Read the model definition and answer for the solid it produces. Units are mm, in the model's axes. Face numbers are marked on the shaded views. A direction names the side the tool comes from. Coordinates: 2 decimals unless noted, no trailing zeros. Loops run counter-clockwise (first coordinate to the right, second up) from the corner with the lowest first, then second, coordinate; pieces in that order, holes last.
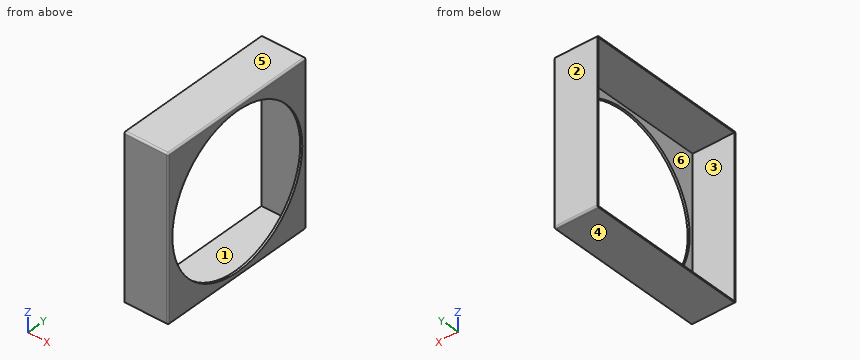
Autodesk Inventor part; units mm, degrees
ref_plane "YZ Plane" through (0, 0, 0) normal (1, 0, 0) x (0, 1, 0)
ref_plane "XZ Plane" through (0, 0, 0) normal (0, 1, 0) x (-1, 0, 0)
ref_plane "XY Plane" through (0, 0, 0) normal (0, 0, 1) x (1, 0, 0)
sketch "Sketch1" plane through (0, 0, 0) normal (1, 0, 0) x (0, 1, 0)
  circle A0 centre (0, 0) radius 139.7
  line L0 (0, -139.7) -> (0, -146.05)
  line L1 (-139.7, 0) -> (-146.05, 0)
  line L2 (146.05, 0) -> (146.05, -146.05)
  line L3 (146.05, -146.05) -> (-146.05, -146.05)
  line L4 (-146.05, -146.05) -> (-146.05, 146.05)
  line L5 (-146.05, 146.05) -> (146.05, 146.05)
  line L6 (146.05, 146.05) -> (146.05, 0)
  dimension "d1" = 279.4
sketch "Sketch2" plane through (0, 0, 0) normal (0, 0, 1) x (1, 0, 0)
  point P0 (0, 0)
extrude "Extrusion1" add sketch "Sketch1" along normal blind 3.81 contours A0 L1 L4 L5 L6 L2 L3 L0 | A0 L0 L3 L4 L1
sketch "Sketch3" plane through (0, -146.05, 146.05) normal (0, 0, 1) x (1, 0, 0)
  line L0 (0, 292.1) -> (0, 0)
  line L1 (3.81, 292.1) -> (-76.2, 292.1)
  line L2 (-76.2, 292.1) -> (-76.2, 0)
  line L3 (-76.2, 0) -> (3.81, 0)
  point P0 (0, 146.05)
  dimension "d12" = 80.01
extrude "Extrusion3" add sketch "Sketch3" along normal blind 2.54
sketch "Sketch4" plane through (3.81, -146.05, -146.05) normal (0, -1, 0) x (1, 0, 0)
  line L0 (-3.81, 292.1) -> (0, 292.1)
  line L1 (-3.81, 292.1) -> (-80.01, 292.1)
  line L2 (-3.81, 292.1) -> (-80.01, 292.1)
  line L3 (-3.81, 292.1) -> (-3.81, 0)
  line L4 (-3.81, 0) -> (-80.01, 0)
  line L5 (-80.01, 0) -> (-80.01, 292.1)
  point P0 (-3.81, 146.05)
  dimension "d15" = 76.2
extrude "Extrusion4" add sketch "Sketch4" along normal blind 2.54
sketch "Sketch6" plane through (3.81, -146.05, -146.05) normal (0, 0, -1) x (-1, 0, 0)
  line L0 (80.01, 0) -> (3.81, 0)
  line L1 (3.81, 0) -> (80.01, 0)
  line L2 (80.01, 292.1) -> (80.01, 0)
  line L3 (80.01, 0) -> (80.01, 292.1)
  line L4 (80.01, 292.1) -> (3.81, 292.1)
  line L5 (3.81, 292.1) -> (3.81, 0)
  line L6 (3.81, 6.35) -> (3.81, 285.75)
  point P0 (3.81, 146.05)
extrude "Extrusion5" add sketch "Sketch6" along normal blind 2.54
sketch "Sketch7" plane through (3.81, 146.05, 146.05) normal (0, 1, 0) x (1, 0, 0)
  line L0 (-3.81, 292.1) -> (0, 292.1)
  line L1 (-3.81, 292.1) -> (-80.01, 292.1)
  line L2 (-80.01, 292.1) -> (-80.01, 0)
  line L3 (-80.01, 0) -> (-3.81, 0)
  line L4 (-3.81, 292.1) -> (-3.81, 0)
  point P0 (-3.81, 146.05)
extrude "Extrusion6" add sketch "Sketch7" along normal blind 2.54
sketch "Sketch21" plane through (-76.2, -148.59, -146.05) normal (-1, 0, 0) x (0, 0, 1)
  line L0 (0, 0) -> (-2.54, 0)
  line L1 (-2.54, 0) -> (-2.54, 2.54)
  line L2 (0, 2.54) -> (-2.54, 2.54)
  line L3 (-2.54, 2.54) -> (0, 2.54)
  line L4 (0, 2.54) -> (0, 0)
  line L5 (0, 2.54) -> (0, 0)
  point P0 (146.05, 148.59)
extrude "Extrusion16" add sketch "Sketch21" against normal up to surface (76.2 mm away)
sketch "Sketch22" plane through (3.81, 148.59, 146.05) normal (0, 1, 0) x (1, 0, 0)
  line L0 (-3.81, 0) -> (-3.81, 294.64)
  line L1 (-80.01, 292.1) -> (-3.81, 292.1)
  line L2 (-3.81, 294.64) -> (-3.81, 292.1)
  line L3 (0, 292.1) -> (0, 0)
  line L4 (-3.81, 292.1) -> (0, 292.1)
  line L5 (0, 292.1) -> (0, 294.64)
  line L6 (0, 294.64) -> (-3.81, 294.64)
  point P0 (-3.81, 146.05)
extrude "Extrusion17" add sketch "Sketch22" against normal up to surface (297.18 mm away)
sketch "Sketch23" plane through (-76.2, -146.05, -146.05) normal (-1, 0, 0) x (0, 0, 1)
  line L0 (0, 292.1) -> (-2.54, 292.1)
  line L1 (-2.54, 292.1) -> (0, 292.1)
  line L2 (292.1, 294.64) -> (0, 294.64)
  line L3 (0, 292.1) -> (0, 294.64)
  line L4 (-2.54, 294.64) -> (-2.54, -2.54)
  line L5 (0, 294.64) -> (-2.54, 294.64)
  line L6 (-2.54, 294.64) -> (-2.54, 292.1)
  point P0 (146.05, 146.05)
extrude "Extrusion18" add sketch "Sketch23" against normal up to surface (76.2 mm away)
sketch "Sketch26" plane through (0, -146.05, 148.59) normal (0, 0, 1) x (1, 0, 0)
  line L0 (0, 292.1) -> (3.81, 292.1)
  line L1 (3.81, 292.1) -> (0, 292.1)
  line L2 (0, 292.1) -> (0, 294.64)
  line L3 (0, 292.1) -> (0, 294.64)
  line L4 (0, 294.64) -> (3.81, 294.64)
  line L5 (3.81, 294.64) -> (3.81, 292.1)
  point P0 (0, 146.05)
extrude "Extrusion20" add sketch "Sketch26" against normal up to surface (294.64 mm away)
sketch "Sketch27" plane through (0, -146.05, 148.59) normal (0, 0, 1) x (1, 0, 0)
  line L0 (0, 0) -> (3.81, 0)
  line L1 (3.81, 0) -> (0, 0)
  line L2 (0, 0) -> (0, -2.54)
  line L3 (0, 0) -> (0, -2.54)
  line L4 (0, -2.54) -> (3.81, -2.54)
  line L5 (0, -2.54) -> (3.81, -2.54)
  line L6 (3.81, 0) -> (3.81, -2.54)
  line L7 (3.81, -2.54) -> (3.81, 0)
  point P0 (0, 146.05)
extrude "Extrusion21" add sketch "Sketch27" against normal up to surface (294.64 mm away)
sketch "Sketch28" plane through (0, 146.05, 148.59) normal (0, -1, 0) x (1, 0, 0)
  line L0 (3.81, 0) -> (3.81, -2.54)
  line L1 (3.81, 0) -> (3.81, -2.54)
  line L2 (3.81, -2.54) -> (0, -2.54)
  line L3 (0, -2.54) -> (0, 0)
  line L4 (0, 0) -> (3.81, 0)
  point P0 (0, -148.59)
extrude "Extrusion22" add sketch "Sketch28" along normal up to surface (292.1 mm away)
sketch "Sketch29" plane through (-76.2, -146.05, -146.05) normal (-1, 0, 0) x (0, 0, 1)
  line L0 (292.1, 292.1) -> (294.64, 292.1)
  line L1 (294.64, 292.1) -> (292.1, 292.1)
  line L2 (292.1, 292.1) -> (292.1, 294.64)
  line L3 (292.1, 292.1) -> (292.1, 294.64)
  line L4 (294.64, 294.64) -> (294.64, 292.1)
  line L5 (292.1, 294.64) -> (294.64, 294.64)
  line L6 (294.64, 294.64) -> (294.64, 292.1)
  point P0 (146.05, 146.05)
extrude "Extrusion23" add sketch "Sketch29" against normal up to surface (76.2 mm away)
sketch "Sketch30" plane through (-76.2, -146.05, -146.05) normal (-1, 0, 0) x (0, 0, 1)
  line L0 (292.1, 0) -> (0, 0)
  line L1 (292.1, 0) -> (292.1, -2.54)
  line L2 (294.64, -2.54) -> (-2.54, -2.54)
  line L3 (294.64, -2.54) -> (294.64, 0)
  line L4 (294.64, -2.54) -> (294.64, 294.64)
  line L5 (292.1, 0) -> (294.64, 0)
  line L6 (292.1, 0) -> (292.1, -2.54)
  line L7 (292.1, -2.54) -> (294.64, -2.54)
  point P0 (146.05, 146.05)
extrude "Extrusion24" add sketch "Sketch30" against normal up to surface (76.2 mm away)
fillet "Fillet1" radius 3.175 8 edges at (-36.195, -148.59, 148.59) (-36.195, -148.59, -148.59) (-36.195, 148.59, -148.59) (-36.195, 148.59, 148.59) (3.81, 148.59, 0) (3.81, 0, 148.59) (3.81, 0, -148.59) (3.81, -148.59, 0)
properties part number "Base box"
Item 1: Find the intervals of material crossed by line 1 along Z through (x, y) = (0.95, 0); line 2 along Y through (x, z) = (-39, 89), in increasing order.
Numbers:
line 1: z = -148.57 to -139.7, 139.7 to 148.57
line 2: y = -148.59 to -146.05, 146.05 to 148.59
Item 2: Which of the six approach directions +Z, -Z, +X, -X, +Y, -Y give full straight-line access (tool end or side, diameter ignored) to the marked faces 5 and 6?
Numbers:
face 5: +Z, +X, -X, +Y, -Y
face 6: -X
Item 3: A cutting plane is placed at A-A on z = 0. Determine the outline of the cut face in (x, y) (3 decimals), then the cut area to 3 significant figures.
Numbers:
outline: (-76.2, -148.59) - (0.635, -148.59) arc R3.175 ccw to (3.81, -145.415) - (3.81, -139.7) - (0, -139.7) - (0, -146.05) - (-76.2, -146.05) - close; (-76.2, 146.05) - (0, 146.05) - (0, 139.7) - (3.81, 139.7) - (3.81, 145.415) arc R3.175 ccw to (0.635, 148.59) - (-76.2, 148.59) - close
area: 451 mm2
Item 4: Determine the mould class of the marked faces 1, 2, 3 and 4 for opening direction Y: released by +Y, released by -Y, zero draft, split by the parting line, or undercut.
Numbers:
face 1: undercut
face 2: released by +Y
face 3: undercut
face 4: zero draft
Item 5: A cutting plane is placed at B-B on y = -59. Determine the outline of the cut face in (x, z) (3 decimals).
Numbers:
outline: (-76.2, -148.59) - (0.635, -148.59) arc R3.175 ccw to (3.81, -145.415) - (3.81, -126.63) - (0, -126.63) - (0, -146.05) - (-76.2, -146.05) - close; (-76.2, 146.05) - (0, 146.05) - (0, 126.63) - (3.81, 126.63) - (3.81, 145.415) arc R3.175 ccw to (0.635, 148.59) - (-76.2, 148.59) - close
Item 6: A cutting plane is placed at C-C on x = -43. Determine the outline of the cut face in (y, z) (3 decimals).
Numbers:
outline: (-148.59, -145.415) arc R3.175 ccw to (-145.415, -148.59) - (145.415, -148.59) arc R3.175 ccw to (148.59, -145.415) - (148.59, 145.415) arc R3.175 ccw to (145.415, 148.59) - (-145.415, 148.59) arc R3.175 ccw to (-148.59, 145.415) - close; hole (-146.05, -146.05) - (146.05, -146.05) - (146.05, 146.05) - (-146.05, 146.05) - close
